Work out the finished part from the listing and answer in its coordinate system (mm). A direction names the side the tool comes from. Coordinates: 2 decimals unless noted, no trailing zeros. Write each loop counter-clockwise with the first axis right and the second up, starting at its lowest first coordinate (ties: lowest second). Pieces come first, ordered by that corner, then holes. Notation, with made-up numbers: (-31.75, 4.5) - (-10.75, 4.5) arc R24 ccw to (-10.75, 28.5) - close; hole circle Ø11 at (45.25, 47). An arc over 180 degrees is marked (long way). Use a Markdown table: item, result. Add a question column.
(1) Given pin 1 Ø2 at (x, z) = (-2, 11) entering from +Y; pin 2 Ø10 at (y, z) = (-5.5, 30.5) entering from -X; pin 3 Ø2 at (y, z) = (2, 40) entering from +X; pin 4 Ø0.6 at (x, z) = (-9, -1.5) entering from +Y, each flat-ended and moving along its own axis, determine where each tip first touches the part or whether it passes through.
(2) The part is cut by section C-C, the plane z = 23. Give the vertices of the cut face in (x, y).
(3) The part is cut by section B-B, the plane y = 9.25. Give the vertices of the cut face in (x, z), then the cut area to 4 significant figures.
(4) A tool of negligible diameter and unlimited length cuts with its end or side. For faces 4 (the face through (8, -0.5, 23)), 5 (the face through (6.9, 1.5, -1)), 6 (the face through (-12.1, 1.5, -1)), 7 (the face through (0, -4.5, 47)), 8 (the face through (-11, 3, -9)), from which of +Z, -Z, +X, -X, +Y, -Y can it reach the whole face along a straight path? Write none if from no direction.
(5) The part is cut by section A-A, the plane z = 10. Give the vertices of the cut face in (x, y), then the cut area to 3 significant figures.
(6) For a pull along X with two mould halves and no side action, classify faces 1 (the face through (-8, 3, 39)), 2 (the face through (-9, 3, -2)), 3 (the face through (0.81, -1.25, 49.75)) as released by +X, released by -X, zero draft, split by the parting line, or undercut.
(7) Find the intervals of material crossed by line 1 (Z direction, x = -1, y = -5); line 2 (Z direction, x = -3.5, y = 4); line 3 (X direction, y = 1, z = 35), in increasing order. Write a range as from..to.
Autodesk Inventor part; units mm, degrees
ref_plane "YZ Plane" through (0, 0, 0) normal (1, 0, 0) x (0, 1, 0)
ref_plane "XZ Plane" through (0, 0, 0) normal (0, 1, 0) x (-1, 0, 0)
ref_plane "XY Plane" through (0, 0, 0) normal (0, 0, 1) x (1, 0, 0)
sketch "Sketch1" plane through (0, 0, 0) normal (0, 0, 1) x (1, 0, 0)
  line L0 (15, -7.5) -> (-15, -7.5)
  line L1 (-15, -7.5) -> (-15, 7.5)
  line L2 (-15, 7.5) -> (15, 7.5)
  line L3 (15, 7.5) -> (15, -7.5)
  line L4 (15, -7.5) -> (-15, 7.5) construction
  line L5 (-15, -7.5) -> (15, 7.5) construction
  point P0 (0, 0)
  dimension "d0" = 15
  dimension "d1" = 30
extrude "Extrusion1" add sketch "Sketch1" along normal blind 30
sketch "Sketch2" plane through (0, 0, 30) normal (0, 0, 1) x (1, 0, 0)
  line L0 (15, 7.5) -> (-15, 7.5)
  line L1 (-15, 7.5) -> (-15, -7.5)
  line L2 (-15, -7.5) -> (15, -7.5)
  line L3 (15, -7.5) -> (15, 7.5)
  circle A0 centre (0, -1) radius 2.5
  point P0 (0, 0)
  dimension "d4" = 6.5
  dimension "d5" = 5
extrude "Extrusion2" add sketch "Sketch2" along normal blind 3.3 contours A0
sketch "Sketch3" plane through (0, -1, 33.3) normal (0, 0, 1) x (1, 0, 0)
  circle A0 centre (0, 0) radius 2.5
  line L0 (-8, 15) -> (8, 15)
  line L1 (8, 15) -> (8, -8)
  line L2 (8, -8) -> (-8, -8)
  line L3 (-8, -8) -> (-8, 15)
  line L4 (-8, 15) -> (8, -8) construction
  line L5 (8, 15) -> (-8, -8) construction
  line L6 (-15, -6.5) -> (15, -6.5)
  point P0 (0, 1)
  point P1 (0, 3.5)
  point P2 (0, 3.5)
  point P3 (-8, -6.5)
  point P4 (8, -6.5)
  dimension "d9" = 23
  dimension "d10" = 16
  dimension "d11" = 8
extrude "Extrusion3" add sketch "Sketch3" along normal blind 11.5 contours A0 | L0 L1 L6 L3
sketch "Sketch4" plane through (-15, -7.5, 0) normal (0, -1, 0) x (1, 0, 0)
  line L0 (0, 0) -> (30, 0)
  line L1 (30, 0) -> (30, 30)
  line L2 (0, 30) -> (30, 30)
  line L3 (0, 0) -> (0, 30)
  circle A0 centre (7, 7) radius 1.4
  circle A1 centre (23, 7) radius 1.4
  circle A2 centre (7, 23) radius 1.4
  circle A3 centre (23, 23) radius 1.4
  point P0 (15, 0)
  point P1 (15, 30)
  dimension "d16" = 16
  dimension "d19" = 16
  dimension "d22" = 8
  dimension "d23" = 7
  dimension "d24" = 2.8
extrude "Extrusion4" cut sketch "Sketch4" against normal blind 7 contours A0 | A1 | A2 | A3
sketch "Sketch5" plane through (0, -1, 44.8) normal (0, 0, 1) x (1, 0, 0)
  circle A0 centre (0, 0) radius 2.5
  line L0 (-2.0207, 3.5) -> (2.0207, 3.5)
  line L1 (2.0207, 3.5) -> (4.0415, 0)
  line L2 (4.0415, 0) -> (2.0207, -3.5)
  line L3 (2.0207, -3.5) -> (-2.0207, -3.5)
  line L4 (-2.0207, -3.5) -> (-4.0415, 0)
  line L5 (-4.0415, 0) -> (-2.0207, 3.5)
  point P0 (0, 1)
  dimension "d35" = 7
extrude "Extrusion5" add sketch "Sketch5" along normal blind 3.3 contours A0 | L0 L1 L2 L3 L4 L5
sketch "Sketch6" plane through (0, -1, 48.1) normal (0, 0, 1) x (1, 0, 0)
  line L0 (-4.0415, 0) -> (-2.0207, -3.5)
  line L1 (-2.0207, -3.5) -> (2.0207, -3.5)
  line L2 (2.0207, -3.5) -> (4.0415, 0)
  line L3 (4.0415, 0) -> (2.0207, 3.5)
  line L4 (2.0207, 3.5) -> (-2.0207, 3.5)
  line L5 (-2.0207, 3.5) -> (-4.0415, 0)
  circle A0 centre (0, 0) radius 2.5
  point P0 (0, 1)
extrude "Extrusion6" add sketch "Sketch6" along normal blind 2 contours A0
chamfer "Chamfer1" distance 2 angle 45 1 edges at (-2.5, -1, 50.1)
sketch "Sketch7" plane through (0, -1, 44.8) normal (0, 0, 1) x (1, 0, 0)
  circle A0 centre (0, 0) radius 2.5
  circle A1 centre (0, 0) radius 2.5
  line L0 (-4.0415, 0) -> (-2.0207, -3.5)
  line L1 (-2.0207, -3.5) -> (2.0207, -3.5)
  line L2 (2.0207, -3.5) -> (4.0415, 0)
  line L3 (4.0415, 0) -> (2.0207, 3.5)
  line L4 (2.0207, 3.5) -> (-2.0207, 3.5)
  line L5 (-2.0207, 3.5) -> (-4.0415, 0)
  point P0 (0, 1)
extrude "Extrusion7" cut sketch "Sketch7" along normal blind 1
chamfer "Chamfer2" distance 2 angle 45 2 edges at (-15, 7.5, 15) (15, 7.5, 15)
chamfer "Chamfer3" distance 0.5 angle 45 22 edges at (-8, 3.25, 33.3) (8, 3.25, 33.3) (0, 14, 33.3) (8, 14, 39.05) (-8, 14, 39.05) (0, 14, 44.8) (-8, 3.25, 44.8) (-8, -7.5, 39.05) (0, -7.5, 33.3) (8, -7.5, 39.05) (0, -7.5, 44.8) (8, 3.25, 44.8) (0, 7.5, 30) (15, -1, 30) (14, 6.5, 30) (-15, -1, 30) (-14, 6.5, 30) (-15, -1, 0) (-14, 6.5, 0) (0, 7.5, 0) (14, 6.5, 0) (15, -1, 0)
sketch "Sketch8" plane through (0, 0, 0) normal (0, 0, -1) x (-1, 0, 0)
  line L0 (-14.5, -7.5) -> (-14.5, 5.2929)
  line L1 (14.5, -7.5) -> (-14.5, -7.5)
  line L2 (14.5, 5.2929) -> (14.5, -7.5)
  line L3 (12.7929, 7) -> (14.5, 5.2929)
  line L4 (-12.7929, 7) -> (12.7929, 7)
  line L5 (-14.5, 5.2929) -> (-12.7929, 7)
  line L6 (7.7679, 6) -> (11.2321, 6)
  line L7 (11.2321, 6) -> (12.9641, 3)
  line L8 (12.9641, 3) -> (11.2321, 0)
  line L9 (11.2321, 0) -> (7.7679, 0)
  line L10 (7.7679, 0) -> (6.0359, 3)
  line L11 (6.0359, 3) -> (7.7679, 6)
  line L12 (-11.2321, 6) -> (-7.7679, 6)
  line L13 (-7.7679, 6) -> (-6.0359, 3)
  line L14 (-6.0359, 3) -> (-7.7679, 0)
  line L15 (-7.7679, 0) -> (-11.2321, 0)
  line L16 (-11.2321, 0) -> (-12.9641, 3)
  line L17 (-12.9641, 3) -> (-11.2321, 6)
  point P0 (0, 0)
  point P1 (9.5, 3)
  point P2 (-9.5, 3)
  dimension "d51" = 6
  dimension "d52" = 5
  dimension "d53" = 5
  dimension "d54" = 4
extrude "Extrusion8" add sketch "Sketch8" along normal blind 2 contours L6 L7 L8 L9 L10 L11 | L12 L13 L14 L15 L16 L17
sketch "Sketch9" plane through (0, 0, -2) normal (0, 0, -1) x (-1, 0, 0)
  line L0 (6.0359, 3) -> (7.7679, 0)
  line L1 (7.7679, 0) -> (11.2321, 0)
  line L2 (11.2321, 0) -> (12.9641, 3)
  line L3 (12.9641, 3) -> (11.2321, 6)
  line L4 (11.2321, 6) -> (7.7679, 6)
  line L5 (7.7679, 6) -> (6.0359, 3)
  line L6 (-12.9641, 3) -> (-11.2321, 0)
  line L7 (-11.2321, 0) -> (-7.7679, 0)
  line L8 (-7.7679, 0) -> (-6.0359, 3)
  line L9 (-6.0359, 3) -> (-7.7679, 6)
  line L10 (-7.7679, 6) -> (-11.2321, 6)
  line L11 (-11.2321, 6) -> (-12.9641, 3)
  circle A0 centre (9.5, 3) radius 1.75
  circle A1 centre (-9.5, 3) radius 1.75
  circle A2 centre (9.5, 3) radius 1
  circle A3 centre (-9.5, 3) radius 1
  point P0 (0, 0)
  point P1 (9.5, 0)
  point P2 (-9.5, 0)
  dimension "d57" = 3.5
  dimension "d58" = 2
extrude "Extrusion9" add sketch "Sketch9" along normal blind 7 contours A0 | A1
sketch "Sketch10" plane through (0, 0, 0) normal (0, 0, -1) x (-1, 0, 0)
  line L0 (-12.9641, 3) -> (-11.2321, 6)
  line L1 (-11.2321, 6) -> (-7.7679, 6)
  line L2 (-7.7679, 6) -> (-6.0359, 3)
  line L3 (-6.0359, 3) -> (-7.7679, 0)
  line L4 (-7.7679, 0) -> (-11.2321, 0)
  line L5 (-11.2321, 0) -> (-12.9641, 3)
  line L6 (6.0359, 3) -> (7.7679, 6)
  line L7 (7.7679, 6) -> (11.2321, 6)
  line L8 (11.2321, 6) -> (12.9641, 3)
  line L9 (12.9641, 3) -> (11.2321, 0)
  line L10 (11.2321, 0) -> (7.7679, 0)
  line L11 (7.7679, 0) -> (6.0359, 3)
  line L12 (-14.5, -7.5) -> (-14.5, 5.2929)
  line L13 (14.5, -7.5) -> (-14.5, -7.5)
  line L14 (14.5, 5.2929) -> (14.5, -7.5)
  line L15 (12.7929, 7) -> (14.5, 5.2929)
  line L16 (-12.7929, 7) -> (12.7929, 7)
  line L17 (-14.5, 5.2929) -> (-12.7929, 7)
  circle A0 centre (0, -1) radius 2.5
  circle A1 centre (0, -1) radius 0.5
  circle A2 centre (0, -1) radius 5
  point P0 (0, 0)
  dimension "d61" = 10
extrude "Extrusion10" add sketch "Sketch10" along normal blind 15 contours A0 | A1 | A2
properties part number "Arethusa" material "Aluminum 6061"
Model answer:
| question | item | result |
|---|---|---|
| 1 | pin 1 | y = 7.5 |
| 1 | pin 2 | x = -15 |
| 1 | pin 3 | x = 8 |
| 1 | pin 4 | y = 6 |
| 2 | outline | (-15, -7.5) - (-9.4, -7.5) - (-9.4, -0.5) - (-6.6, -0.5) - (-6.6, -7.5) - (6.6, -7.5) - (6.6, -0.5) - (9.4, -0.5) - (9.4, -7.5) - (15, -7.5) - (15, 5.5) - (13, 7.5) - (-13, 7.5) - (-15, 5.5) - close |
| 3 | outline | (-8, 33.8) - (-7.5, 33.3) - (7.5, 33.3) - (8, 33.8) - (8, 44.3) - (7.5, 44.8) - (-7.5, 44.8) - (-8, 44.3) - close |
| 3 | area | 183.5 mm^2 |
| 4 | face 4 | -Y |
| 4 | face 5 | -Z, -Y |
| 4 | face 6 | -Z, -X, -Y |
| 4 | face 7 | +Z, +X, -X, -Y |
| 4 | face 8 | -Z, -X, +Y, -Y |
| 5 | outline | (-15, -7.5) - (15, -7.5) - (15, 5.5) - (13, 7.5) - (-13, 7.5) - (-15, 5.5) - close |
| 5 | area | 446 mm^2 |
| 6 | face 1 | released by -X |
| 6 | face 2 | undercut |
| 6 | face 3 | split by the parting line |
| 7 | line 1 | -15..30, 33.3..44.8 |
| 7 | line 2 | 0..30, 33.3..44.8 |
| 7 | line 3 | -8..8 |
